CAD build for the part. Positions are in the model's coordinates, mm. A direction names the side the tool comes from. Round coordinates to 2 decimals unless told otherwise and drop trailing zeros. Order: outer loops, then holes, each group sorted by start corner. A loop starts at its lowest first (then second) coordinate and runs counter-clockwise, first axis right, second up. Notation, with made-up numbers: (14, 65.5) - (38, 65.5) arc R12 ccw to (38, 85.5) - close; hole circle Ø10 at (-27.5, 52.25). An arc over 180 degrees is marked (long way). Write item = value, one per line.
from build123d import *

# Parameters (mm, degrees)
CHAMFER1_SIZE      = 0.8
CUT_EXTRUDE1_DEPTH = 6


with BuildPart() as part:
    # Sketch1 → Revolve1 (revolve)
    with BuildSketch(Plane(origin=(0, 0, 0), x_dir=(0, 0, -1), z_dir=(1, 0, 0))):
        Polygon((0, 0), (0, 6.5), (0.53, 7.417986928), (8.53, 7.417986928), (9.06, 6.5), (9.06, 4), (39.06, 4), (39.06, 0), align=None)
    revolve(axis=Axis((0, 0, 0), (0, 0, -1)))

    # Chamfer1
    chamfer1_edges = [part.edges().sort_by_distance(p)[0] for p in [
        (0, -4, -39.06),
    ]]
    chamfer(chamfer1_edges, length=CHAMFER1_SIZE)

    # Sketch2 → Cut-Extrude1 (cut)
    with BuildSketch(Plane.XY):
        Polygon((3.25, -1.876388375), (3.25, 1.876388375), (0, 3.75277675), (-3.25, 1.876388375), (-3.25, -1.876388375), (0, -3.75277675), align=None)
    extrude(amount=-CUT_EXTRUDE1_DEPTH, mode=Mode.SUBTRACT)

    # Sketch3 → Cut-Revolve1 (revolve, cut)
    with BuildSketch(Plane(origin=(0, 0, 0), x_dir=(0, 0, -1), z_dir=(1, 0, 0))):
        Polygon((0, 0), (0, 4), (2.309401077, 0), align=None)
        Polygon((8.166666667, 0), (6, 0), (6, 3.75277675), align=None)
    revolve(axis=Axis((0, 0, 0), (0, 0, -1)), mode=Mode.SUBTRACT)


solid = part.part
(1) Band-saw the part on A-A on z = -5. List the corners of the cut face in (x, y), plus the area to 3 significant figures.
Solved:
outline = circle Ø14.84 at (0, 0); hole (-3.25, -1.88) - (0, -3.75) - (3.25, -1.88) - (3.25, 1.88) - (0, 3.75) - (-3.25, 1.88) - close
area = 136 mm²
(2) Band-saw the part on B-B on z = -30. List the corners of the cut face in (x, y), plus the area to 3 significant figures.
Solved:
outline = circle Ø8 at (0, 0)
area = 50.3 mm²
(3) Probe line 1 along Z through (x, y) = (-4.75, -2); line 2 along X through (y, z) = (-2.5, -4.5); line 3 along X through (y, z) = (-0.25, -26.5). List the from-to ranges inside material, lowest first.
Solved:
line_1 = -9.06 to 0
line_2 = -6.98 to -2.17, 2.17 to 6.98
line_3 = -3.99 to 3.99
(4) Drop flat-ended pins along their axis: pin 1 (1 mm diameter, centred on y = 1, z = -25, fed in from -X); pin 2 (8 mm diameter, centred on y = -2, z = -34, fed in from +X); pin 3 (3 mm diameter, centred on x = 4, z = -18.5, fed in from -Y). Give the stop position or say it passes through.
Solved:
pin_1 = -3.97
pin_2 = 4
pin_3 = -3.12
(5) Tool access for faces 1 (the flat face through (-1.7, 3, -6)), 2 (the flat face through (0, 0, -39.06)), 3 (the flat face through (-3.25, 0, -3)), 4 (the cylindrical face through (-3.905, -0.867, -23.864)): list every direction of +Z, -Z, +X, -X, +Y, -Y with a clear straight run to the whole face (end or side of a thin tool).
Solved:
face_1 = none
face_2 = -Z, +X, -X, +Y, -Y
face_3 = +Z
face_4 = -Z
(6) Pull direction Z, two halves, no side cores. Call faces 5 (the flat face through (3, -3, 0)), 6 (the flat face through (-1.6, 2.83, -3.03)), 7 (the flat face through (1.63, -3.02, -6)): released by +Z, released by -Z, zero draft, split by the parting line, or undercut.
Solved:
face_5 = released by +Z
face_6 = zero draft
face_7 = undercut
